Could you check a few things on this model? Use its own coordinates, in mm. Coordinates: 2 decimals unless noted, no trailing zeros. Order: outer loops, then holes, each group sorted by start corner. A loop starts at its lowest first (then second) coordinate and runs counter-clockwise, first axis right, second up. Notation, with made-up numbers: (52.5, -33.75) - (98.5, -33.75) arc R5 cw to (98.5, -25.75) - close; hole circle Ø9 at (28.25, 54). An arc over 180 degrees is marked (long way). Answer as a JSON object with one key per item and string values. Group by question number.
(1) Imagine slicing it at A-A, the plane z = 40. Write out the boundary of the cut face in (x, y) (3 decimals), and give its area (3 significant figures).
(2) Please list where these lines run through material, in increasing order: probe 1 along Z at (x, y) = (-26, -2); probe 2 along Z at (x, y) = (14, -2.9); probe 3 along X at (y, z) = (-2.6, 23) (3 decimals).
(3) Imagine slicing it at D-D, the plane z = 17.5. Write out the boundary of the cut face in (x, y) (3 decimals), and give its area (3 significant figures).
(4) Will these pins go through, and if not, where does the flat tip stop? P1, Ø3.5, axis at x = -17.23, z = 93.98, coming from the -Y side (3 decimals); P2, Ø1.7, axis at x = 13.76, z = 93.98, coming from the +Y side.
(5) Imagine slicing it at C-C, the plane y = -0.55. Write out the boundary of the cut face in (x, z) (3 decimals).
(6) Imagine slicing it at B-B, the plane x = -10. Write out the boundary of the cut face in (y, z) (3 decimals).
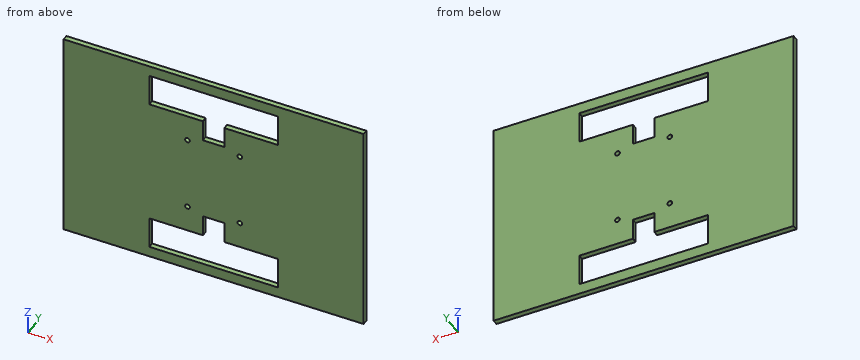
from build123d import *

# Parameters (mm, degrees)
F0_W     = 177.8
F0_H     = 127
F0_R     = 1.397
F1_DEPTH = 3.175


# Not quite as in the source:
# - a feature names something its author has since deleted; it is built from what else it names


with BuildPart() as f1:
    # F0 (on Front) → F1 (new body)
    with BuildSketch(Plane.XZ):
        with Locations((-1.7349944949, 71.7831266678)):
            Rectangle(F0_W, F0_H)
        with Locations((-17.2289944949, 49.5835266678)):
            Circle(F0_R, mode=Mode.SUBTRACT)
        Polygon((-39.8349944949, 14.6331266678), (-39.8349944949, 33.6831266678), (-8.0849944949, 33.6831266678), (-8.0849944949, 46.3831266678), (4.6150055051, 46.3831266678), (4.6150055051, 33.6831266678), (36.3650055051, 33.6831266678), (36.3650055051, 14.6331266678), align=None, mode=Mode.SUBTRACT)
        with Locations((13.7590055051, 49.5835266678)):
            Circle(F0_R, mode=Mode.SUBTRACT)
        with Locations((-17.2289944949, 93.9827266678)):
            Circle(F0_R, mode=Mode.SUBTRACT)
        Polygon((-39.8349944949, 109.8831266678), (-39.8349944949, 128.9331266678), (36.3650055051, 128.9331266678), (36.3650055051, 109.8831266678), (4.6150055051, 109.8831266678), (4.6150055051, 97.1831266678), (-8.0849944949, 97.1831266678), (-8.0849944949, 109.8831266678), align=None, mode=Mode.SUBTRACT)
        with Locations((13.7590055051, 93.9827266678)):
            Circle(F0_R, mode=Mode.SUBTRACT)
    extrude(amount=F1_DEPTH)


solid = f1.part
Result set:
{
 "1": {"outline": "(-90.635, -3.175) - (-8.085, -3.175) - (-8.085, 0) - (-90.635, 0) - close; (4.615, -3.175) - (87.165, -3.175) - (87.165, 0) - (4.615, 0) - close", "area": "524 mm^2"},
 "2": {"probe 1": "z = 8.28 to 14.63, 33.68 to 109.88, 128.93 to 135.28", "probe 2": "z = 8.28 to 14.63, 33.68 to 48.21, 50.96 to 92.61, 95.36 to 109.88, 128.93 to 135.28", "probe 3": "x = -90.635 to -39.835, 36.365 to 87.165"},
 "3": {"outline": "(-90.635, -3.175) - (-39.835, -3.175) - (-39.835, 0) - (-90.635, 0) - close; (36.365, -3.175) - (87.165, -3.175) - (87.165, 0) - (36.365, 0) - close", "area": "323 mm^2"},
 "4": {"P1": "stops at y = -3.175", "P2": "passes through"},
 "5": {"outline": "(-90.635, 8.283) - (87.165, 8.283) - (87.165, 135.283) - (-90.635, 135.283) - close; hole (-39.835, 14.633) - (36.365, 14.633) - (36.365, 33.683) - (4.615, 33.683) - (4.615, 46.383) - (-8.085, 46.383) - (-8.085, 33.683) - (-39.835, 33.683) - close; hole (-39.835, 109.883) - (-8.085, 109.883) - (-8.085, 97.183) - (4.615, 97.183) - (4.615, 109.883) - (36.365, 109.883) - (36.365, 128.933) - (-39.835, 128.933) - close; hole circle Ø2.794 at (-17.229, 49.584); hole circle Ø2.794 at (-17.229, 93.983); hole circle Ø2.794 at (13.759, 49.584); hole circle Ø2.794 at (13.759, 93.983)"},
 "6": {"outline": "(-3.175, 8.283) - (0, 8.283) - (0, 14.633) - (-3.175, 14.633) - close; (-3.175, 33.683) - (0, 33.683) - (0, 109.883) - (-3.175, 109.883) - close; (-3.175, 128.933) - (0, 128.933) - (0, 135.283) - (-3.175, 135.283) - close"}
}
